```python
from build123d import *

# Parameters (mm, degrees)
SKETCH1_R           = 4.445
BOSS_EXTRUDE2_DEPTH = 50.8
SKETCH2_R           = 8.255
CUT_EXTRUDE1_DEPTH  = 141.089519336
SKETCH3_R           = 1.5
CUT_EXTRUDE2_DEPTH  = 141.089519442
SKETCH4_R           = 11.43
SKETCH4_R_2         = 8.89
BOSS_EXTRUDE3_DEPTH = 6.35


with BuildPart() as part:
    # Sketch1 → Boss-Extrude2 (new body)
    with BuildSketch(Plane(origin=(0, 0, 0), x_dir=(1, 0, 0), z_dir=(0, 1, 0))):
        with BuildLine():
            ThreePointArc((-0.8255, -7.575153447), (7.62, 0), (-0.8255, 7.575153447))
            ThreePointArc((-0.8255, 7.575153447), (20.462166579, 48.403489486), (63.5, 64.77))
            Line((63.5, 64.77), (63.5, 69.85))
            ThreePointArc((63.5, 69.85), (15.695186698, 50.928600267), (-6.2103, 4.415492488))
            ThreePointArc((-6.2103, 4.415492488), (-7.62, 0), (-6.2103, -4.415492488))
            ThreePointArc((-6.2103, -4.415492488), (63.5, -69.85), (133.2103, -4.415492488))
            ThreePointArc((133.2103, -4.415492488), (123.143643591, 6.572131712), (127.8255, -7.575153447))
            ThreePointArc((127.8255, -7.575153447), (63.5, -64.77), (-0.8255, -7.575153447))
        make_face()
        with Locations(Location((0, 0, 0), (0, 0, 270))):
            Circle(SKETCH1_R, mode=Mode.SUBTRACT)
        with Locations(Location((127, 0, 0), (0, 0, 270))):
            Circle(SKETCH1_R, mode=Mode.SUBTRACT)
    extrude(amount=BOSS_EXTRUDE2_DEPTH)

    # Sketch2 → Cut-Extrude1 (cut, through all)
    with BuildSketch(Plane(origin=(47.625, 0, -27.49630657), x_dir=(0, -1, 0), z_dir=(-0.8660254037844398, 0, 0.499999999999998))):
        with Locations(Location((-25.4, 31.75, 0), (0, 0, 270))):
            Circle(SKETCH2_R)
    extrude(amount=CUT_EXTRUDE1_DEPTH, mode=Mode.SUBTRACT)

    # Sketch3 → Cut-Extrude2 (cut, through all)
    with BuildSketch(Plane(origin=(47.625, 0, -27.49630657), x_dir=(0, -1, 0), z_dir=(-0.8660254037844398, 0, 0.499999999999998))):
        with Locations(Location((-42.4, 14.75, 0), (0, 0, 270))):
            Circle(SKETCH3_R)
        with Locations(Location((-8.4, 14.75, 0), (0, 0, 270))):
            Circle(SKETCH3_R)
        with Locations(Location((-8.4, 48.75, 0), (0, 0, 270))):
            Circle(SKETCH3_R)
        with Locations(Location((-42.4, 48.75, 0), (0, 0, 270))):
            Circle(SKETCH3_R)
    extrude(amount=CUT_EXTRUDE2_DEPTH, mode=Mode.SUBTRACT)

    # Sketch4 → Boss-Extrude3 (add)
    with BuildSketch(Plane(origin=(-9.567317666, 0, 5.52369343), x_dir=(0, -1, 0), z_dir=(-0.8660254037844398, 0, 0.499999999999998))):
        with Locations(Location((-25.4, 31.75, 0), (0, 0, 90))):
            Circle(SKETCH4_R)
        with Locations(Location((-25.4, 31.75, 0), (0, 0, 90))):
            Circle(SKETCH4_R_2, mode=Mode.SUBTRACT)
    extrude(amount=-BOSS_EXTRUDE3_DEPTH)


solid = part.part
```
Input: part model. Units: mm. Frame: model coordinates. A direction names the side the tool comes from. Coordinates: 2 decimals unless noted, no trailing zeros. Write each loop counter-clockwise with the first axis right and the second up, starting at its lowest first coordinate (ties: lowest second). Pieces come first, ordered by that corner, then holes.
1) Section D-D on x = 21.5. Output: boundary loops of the cut face in (y, z), and give its area (3 significant figures).
2) Section B-B on z = 0. Output: boundary loops of the cut face in (x, y) (3 decimals), and give its area (3 significant figures).
3) Set-up query: faces 1 (the cylindrical face through (9.59, 25.04, 40.65)), 2 (the flat face through (11.78, 16.14, 29.8)), 3 (the flat face through (63.5, 25, -67)). Return all of +Z, -Z, +X, -X, +Y, -Y with unobstructed straight access to the full face (end or side cutting, diameter ignored); none if empty.
4) Mould query, pull axis X, two halves, no side actions, for faces 4 (the flat face through (5, 0, 5)), 5 (the cylindrical face through (-7.62, 25.04, -0.07)), 6 (the cylindrical face through (62.026, 25.044, 69.834)), 7 (the cylindrical face through (131.407, 25.044, -0.579)). Classes: pulls with the +X half, pulls with the -X half, needs draft (parallel to the pull), parting line crosses it, or undercut.
5) Section A-A on y = 30.5. State how many separate pieces and enclosed holes the cut face has, and give its area (3 significant figures).
6) Pin query (flat end, axial travel): pin 1 Ø10 at (x, y) = (111.5, 24) entering from -Z; pin 2 Ø4 at (y, z) = (23.5, -66.5) entering from +X; pin 3 Ø5 at (x, y) = (45, 33) entering from +Z. Return the tip coordinate at first contact, or that it passes through.
7) Material intervals for line 1 along X through (y, z) = (32, 51.5); line 2 along Z through (x, y) = (29, 15); line 3 along Z through (x, y) = (36, 7), sorted ascending.
Check result:
1. outline: (0, -55.81) - (50.8, -55.81) - (50.8, -49.31) - (0, -49.31) - close; (0, 49.31) - (50.8, 49.31) - (50.8, 55.81) - (0, 55.81) - close
1. area: 661 mm2
2. outline: (-7.62, 0) - (-4.445, 0) - (-4.445, 50.8) - (-7.62, 50.8) - close; (4.445, 0) - (7.62, 0) - (7.62, 50.8) - (4.445, 50.8) - close; (119.38, 0) - (122.555, 0) - (122.555, 50.8) - (119.38, 50.8) - close; (131.445, 0) - (134.62, 0) - (134.62, 50.8) - (131.445, 50.8) - close
2. area: 645 mm2
3. face 1: none
3. face 2: +Y, -Y
3. face 3: -Z, +X, +Y, -Y
4. face 4: needs draft
4. face 5: pulls with the -X half
4. face 6: parting line crosses it
4. face 7: undercut
5. separate pieces: 2
5. enclosed holes: 2
5. area: 1,710 mm2
6. pin 1: stops at z = 37.23
6. pin 2: stops at x = 63.5
6. pin 3: stops at z = 67.99
7. line 1: x = 16.31 to 24.22, 102.78 to 110.69
7. line 2: z = -60.74 to -54.82, 54.82 to 60.74
7. line 3: z = -64.21 to -58.64, 58.64 to 64.21
